from build123d import *

# Parameters (mm, degrees)
SKETCH1_W                                    = 19
SKETCH1_H                                    = 30
PLATE_DEPTH                                  = 4.5
SKETCH2_R                                    = 4.5
CYLINDER_DEPTH                               = 14.5
CLEARANCE_START                              = -14.5
SKETCH2_2_R                                  = 4.5
CLEARANCE_DEPTH                              = 15.5
FILLET1_R                                    = 1
CSK_FOR_M4_COUNTERSUNK_FLAT_HEAD_SCR_2_COUNT = 2
CSK_FOR_M4_COUNTERSUNK_FLAT_HEAD_SCR_2_PITCH = 20


with BuildPart() as part:
    # Sketch1 → Plate (new body)
    with BuildSketch(Plane(origin=(0, 0, 0), x_dir=(0, 0, -1), z_dir=(1, 0, 0))):
        with Locations((9.5, 15)):
            Rectangle(SKETCH1_W, SKETCH1_H)
    extrude(amount=PLATE_DEPTH)

    # Sketch2 → Cylinder (add)
    with BuildSketch(Plane(origin=(0, 30, 0), x_dir=(1, 0, 0), z_dir=(0, 1, 0))):
        with Locations((4.5, 0)):
            Circle(SKETCH2_R)
    extrude(amount=-CYLINDER_DEPTH)

    # Sketch2<2> → Clearance (cut)
    with BuildSketch(Plane(origin=(0, 30, 0), x_dir=(1, 0, 0), z_dir=(0, 1, 0)).offset(CLEARANCE_START)):
        with Locations((4.5, 0)):
            Circle(SKETCH2_2_R)
    extrude(amount=-CLEARANCE_DEPTH, mode=Mode.SUBTRACT)

    # Fillet1
    fillet1_edges = [part.edges().sort_by_distance(p)[0] for p in [
        (2.25, 30, -19),
        (2.25, 0, -19),
    ]]
    fillet(fillet1_edges, radius=FILLET1_R)

    # Sketch4 → CSK for M4 Countersunk Flat Head Screw1 (revolve, cut)
    with BuildSketch(Plane(origin=(4.5, 25, -10), x_dir=(0, 0, -1), z_dir=(0, 1, 0))):
        Polygon((0, 0), (0, 4.5), (2.25, 4.5), (2.25, 2.45), (4.7, 0), align=None)
    csk_for_m4_countersunk_flat_head_screw1 = revolve(axis=Axis((10.85, 25, -10), (-1, 0, 0)), mode=Mode.SUBTRACT)

    # CSK for M4 Countersunk Flat Head Scr 2: CSK for M4 Countersunk Flat Head Screw1 ×2
    with Locations(*[(0, -i * CSK_FOR_M4_COUNTERSUNK_FLAT_HEAD_SCR_2_PITCH, 0) for i in range(1, CSK_FOR_M4_COUNTERSUNK_FLAT_HEAD_SCR_2_COUNT)]):
        add(csk_for_m4_countersunk_flat_head_screw1, mode=Mode.SUBTRACT)


solid = part.part
Source: CAD feature listing. Evaluate the final solid. Frame: model axes, mm. A direction names the side the tool comes from. Give positions to 0.01 mm unless a question says otherwise; leave off trailing zeros. Order: outer loops, then holes, each group sorted by start corner. A loop starts at its lowest first (then second) coordinate and runs counter-clockwise, first axis right, second up. Notation, with made-up numbers: (51.25, 54) -> (88.25, 54) arc R21 cw to (88.25, 71) -> close; hole circle Ø6 at (-35.5, -13). An arc over 180 degrees is marked (long way). Write item = value, one per line.
Item 1: Set-up query: faces 4 (the face through (1.353, 7.858, -3.217)), 5 (the face through (1.039, 27.196, -9.512)), 6 (the face through (4.5, 15, -12)). Return all of +Z, -Z, +X, -X, +Y, -Y with unobstructed straight access to the full face (end or side cutting, diameter ignored); none if empty.
Check result:
face_4 = +Z, +X, -Y
face_5 = +X, -X
face_6 = -Z, +X, +Y, -Y
Item 2: Mould query, pull axis Z, two halves, no side actions, for faces 1 (the face through (1.039, 4.901, -7.752)), 2 (the face through (2.282, 0.285, -18.699)), 3 (the face through (4, 15.5, 0)). Classes: +Z half, -Z half, draft (parallel to the pull), parting line (faces both ways), or undercut.
Check result:
face_1 = undercut
face_2 = -Z half
face_3 = draft
Item 3: Section query A-A (y = 25). Output: boundary loops of the cut face in (x, z).
Check result:
outline = (0, -19) -> (4.5, -19) -> (4.5, -14.7) -> (2.05, -12.25) -> (0, -12.25) -> close; (0, -7.75) -> (2.05, -7.75) -> (4.5, -5.3) -> (4.5, -4.5) arc R4.5 ccw (long way) to (0, 0) -> close
Item 4: Contact query for flat-ended pins moving along their axis: pin 1 (5 mm diameter, centred on y = 4, z = -10, fed in from +X); pin 2 (4 mm diameter, centred on y = 12, z = -7, fed in from +X); pin 3 (7 mm diameter, centred on y = 5, z = -10, fed in from -X); pin 4 (2.5 mm diameter, centred on y = 25, z = -10, fed in from +X). Output: stop coordinate, or through.
Check result:
pin_1 = 3.3
pin_2 = 4.5
pin_3 = 0
pin_4 = through
Item 5: Section query D-D (y = 5). Output: boundary loops of the cut face in (x, z).
Check result:
outline = (0, -19) -> (4.5, -19) -> (4.5, -14.7) -> (2.05, -12.25) -> (0, -12.25) -> close; (0, -7.75) -> (2.05, -7.75) -> (4.5, -5.3) -> (4.5, -4.5) arc R4.5 cw to (0, 0) -> close
Item 6: Section query C-C (x = 3.75). Output: boundary loops of the cut face in (y, z), then the cut area to 3 significant figures.
Check result:
outline = (0, -18) arc R1 ccw to (1, -19) -> (29, -19) arc R1 ccw to (30, -18) -> (30, 4.44) -> (15.5, 4.44) -> (15.5, -4.44) -> (0, -4.44) -> close; hole circle Ø7.9 at (5, -10); hole circle Ø7.9 at (25, -10)
area = 467 mm²
Item 7: Section query B-B (z = -10). Output: boundary loops of the cut face in (x, y).
Check result:
outline = (0, 0) -> (4.5, 0) -> (4.5, 0.3) -> (2.05, 2.75) -> (0, 2.75) -> close; (0, 7.25) -> (2.05, 7.25) -> (4.5, 9.7) -> (4.5, 20.3) -> (2.05, 22.75) -> (0, 22.75) -> close; (0, 27.25) -> (2.05, 27.25) -> (4.5, 29.7) -> (4.5, 30) -> (0, 30) -> close
Item 8: Ray query, probe 1 along Y at (x, z) = (1.45, -10); probe 2 along X at (y, z) = (7.75, -17.5); probe 3 along Z at (x, y) = (1, 5). Return the intervals inside material, ascending.
Check result:
probe_1 = 0 to 2.75, 7.25 to 22.75, 27.25 to 30
probe_2 = 0 to 4.5
probe_3 = -19 to -12.25, -7.75 to -2.83
